from build123d import *

# Parameters (mm, degrees)
BOSS_EXTRUDE1_DEPTH      = 26.67
SKETCH3_W                = 40.639965772
SKETCH3_H                = 26.67
BOSS_EXTRUDE2_DEPTH      = 35.56
CUT_EXTRUDE3_START       = 3.81
CUT_EXTRUDE3_DEPTH       = 19.05
SKETCH9_W                = 30.48
SKETCH9_H                = 19.05
CUT_EXTRUDE4_DEPTH       = 35.533627808
CUT_EXTRUDE8_REACH       = 50.855
SKETCH10_R               = 3.429
SKETCH11_R               = 5.715
CUT_EXTRUDE9_DEPTH       = 3.048
SKETCH12_R               = 5.715
CUT_EXTRUDE10_DEPTH      = 3.048
SKETCH13_R               = 5.715
CUT_EXTRUDE11_DEPTH      = 3.048
CUT_EXTRUDE12_DEPTH      = 49.855187132
CUT_EXTRUDE12_DEPTH_BACK = 49.855187132
SKETCH16_R               = 3.429


with BuildPart() as part:
    # Sketch2 → Boss-Extrude1 (new body)
    with BuildSketch(Plane.XY):
        with BuildLine():
            Line((-20.319982886, 0.026372192), (20.319982886, 0.026372192))
            ThreePointArc((20.319982886, 0.026372192), (0, 20.32), (-20.319982886, 0.026372192))
        make_face()
    extrude(amount=BOSS_EXTRUDE1_DEPTH)

    # Sketch3 → Boss-Extrude2 (add)
    with BuildSketch(Plane(origin=(0, 0.026372192, 0), x_dir=(-1, 0, 0), z_dir=(0, -1, 0))):
        with Locations((0, -13.335)):
            Rectangle(SKETCH3_W, SKETCH3_H)
    extrude(amount=BOSS_EXTRUDE2_DEPTH)

    # Sketch8 → Cut-Extrude3 (cut)
    with BuildSketch(Plane.XY.offset(CUT_EXTRUDE3_START)):
        with BuildLine():
            Line((15.24, 0), (-15.24, 0))
            ThreePointArc((-15.24, 0), (0, 15.24), (15.24, 0))
        make_face()
    extrude(amount=CUT_EXTRUDE3_DEPTH, mode=Mode.SUBTRACT)

    # Sketch9 → Cut-Extrude4 (cut)
    with BuildSketch(Plane(origin=(0, 0, 0), x_dir=(1, 0, 0), z_dir=(0, 1, 0))):
        with Locations((0, -13.335)):
            Rectangle(SKETCH9_W, SKETCH9_H)
    extrude(amount=-CUT_EXTRUDE4_DEPTH, mode=Mode.SUBTRACT)

    # Cut-Extrude8: up to this face of the body (flat: up to its plane)
    cut_extrude8_end = Plane(part.part.faces().sort_by_distance((0, -9.587434333, 26.67))[0])
    # Sketch10 → Cut-Extrude8 (cut, up to the picked face)
    with BuildSketch(Plane.XY, mode=Mode.PRIVATE) as cut_extrude8_sk1:
        with Locations(Location((0, 0, 0), (0, 0, 180))):
            Circle(SKETCH10_R)
    cut_extrude8_tool1 = split(extrude(cut_extrude8_sk1.sketch, amount=CUT_EXTRUDE8_REACH, mode=Mode.PRIVATE), bisect_by=cut_extrude8_end, keep=Keep.BOTH, mode=Mode.PRIVATE)
    add(cut_extrude8_tool1.solids().sort_by(Axis((0, 0, 0), (0, 0, 1)))[0], mode=Mode.SUBTRACT)

    # Sketch11 → Cut-Extrude9 (cut)
    with BuildSketch(Plane.XY):
        with Locations(Location((12.7, 0, 0), (0, 0, 180))):
            Circle(SKETCH11_R)
    extrude(amount=CUT_EXTRUDE9_DEPTH, mode=Mode.SUBTRACT)

    # Sketch12 → Cut-Extrude10 (cut)
    with BuildSketch(Plane.XY):
        with Locations(Location((12.7, -25.4, 0), (0, 0, 180))):
            Circle(SKETCH12_R)
    extrude(amount=CUT_EXTRUDE10_DEPTH, mode=Mode.SUBTRACT)

    # Sketch13 → Cut-Extrude11 (cut)
    with BuildSketch(Plane(origin=(0, 0, 0), x_dir=(-1, 0, 0), z_dir=(0, 0, -1))):
        with Locations((12.7, 0)):
            Circle(SKETCH13_R)
        with Locations((12.7, -25.4)):
            Circle(SKETCH13_R)
    extrude(amount=-CUT_EXTRUDE11_DEPTH, mode=Mode.SUBTRACT)

    # Sketch16 → Cut-Extrude12 (cut, two sides: drawn at the far end of the back side and taken through both)
    with BuildSketch(Plane(origin=(0, 0, 0), x_dir=(-1, 0, 0), z_dir=(0, 0, -1)).offset(-CUT_EXTRUDE12_DEPTH_BACK)):
        with Locations((0, -25.4)):
            Circle(SKETCH16_R)
    extrude(amount=CUT_EXTRUDE12_DEPTH + CUT_EXTRUDE12_DEPTH_BACK, mode=Mode.SUBTRACT)


solid = part.part
Model file for the job. Use its own axes, mm. A direction names the side the tool comes from. Give positions to 0.01 mm unless a question says otherwise; leave off trailing zeros. Loops run counter-clockwise (first coordinate to the right, second up) from the corner with the lowest first, then second, coordinate; pieces in that order, holes last. Notation, with made-up numbers: (82, 13.25) - (109, 13.25) arc R22 cw to (109, 26.25) - close; hole circle Ø3 at (77.25, 61.5). An arc over 180 degrees is marked (long way). Use one line per item in the form item = value.
(1) Cut at A-A (y = -25.4). Give the cut face in (x, z) (3 decimals), then the cut area to 3 significant figures.
Determined:
outline = (-20.32, 0) - (-18.415, 0) - (-18.415, 3.048) - (-6.985, 3.048) - (-6.985, 0) - (-3.429, 0) - (-3.429, 3.81) - (-15.24, 3.81) - (-15.24, 22.86) - (-3.429, 22.86) - (-3.429, 26.67) - (-20.32, 26.67) - close; (3.429, 0) - (6.985, 0) - (6.985, 3.048) - (18.415, 3.048) - (18.415, 0) - (20.32, 0) - (20.32, 26.67) - (3.429, 26.67) - (3.429, 22.86) - (15.24, 22.86) - (15.24, 3.81) - (3.429, 3.81) - close
area = 381 mm^2
(2) Drop flat-ended pins along their axis: P1, Ø4, axis at x = 0, y = -25.4, coming from the +Z side; P2, Ø2, axis at x = 10, z = 9.5, coming from the -Y side; P3, Ø6, axis at x = -3, z = 16.5, coming from the +Y side; P4, Ø6, axis at y = 14.5, z = 9, coming from the -X side. Give the stop position or say it passes through.
Determined:
P1 = through
P2 = 10.55
P3 = 20.32
P4 = -16.75
(3) 3-axis set-ups, long thin cutter, end or side, ignore diameter. For faces 4 (the face through (20.32, -18, 14)), 5 (the face through (0, -10, 22.86)), 6 (the face through (13, -25, 3.048)): which of +Z, -Z, +X, -X, +Y, -Y reach the whole face in a straight line?
Determined:
face_4 = +Z, -Z, +X, +Y, -Y
face_5 = -Y
face_6 = -Z
(4) Pull direction Y, two halves, no side cores. Call faces 1 (the face through (0, -35.534, 25)), 2 (the face through (0, -10, 3.81)), 3 (the face through (0.74, 3.35, 24.74)): pulls with the +Y half, pulls with the -Y half, needs draft (parallel to the pull), parting line crosses it, or undercut.
Determined:
face_1 = pulls with the -Y half
face_2 = needs draft
face_3 = undercut
(5) Cut at C-C (y = -13). Give the cut face in (x, z), then the cut area to 3 significant figures.
Determined:
outline = (-20.32, 0) - (20.32, 0) - (20.32, 26.67) - (-20.32, 26.67) - close; hole (-15.24, 3.81) - (15.24, 3.81) - (15.24, 22.86) - (-15.24, 22.86) - close
area = 503 mm^2
(6) Cut at D-D (z = 2.25). Give the cut face in (x, y) (3 decimals), then the cut area to 3 significant figures.
Determined:
outline = (-20.32, -35.534) - (20.32, -35.534) - (20.32, 0.026) arc R20.32 ccw to (-20.32, 0.026) - close; hole circle Ø11.43 at (-12.7, -25.4); hole circle Ø11.43 at (-12.7, 0); hole circle Ø6.858 at (0, -25.4); hole circle Ø6.858 at (0, 0); hole circle Ø11.43 at (12.7, -25.4); hole circle Ø11.43 at (12.7, 0)
area = 1,610 mm^2
(7) Drill centre lines: L1, parallel to Y at x = 0, z = 1.65; L2, parallel to Z at x = 1, y = -13.5; L3, parallel to Z at x = 10, y = 3. Where is each one in solid material? Low to high.
Determined:
L1 = -35.53 to -28.83, -21.97 to -3.43, 3.43 to 20.32
L2 = 0 to 3.81, 22.86 to 26.67
L3 = 3.05 to 3.81, 22.86 to 26.67
(8) Cut at B-B (x = 0). Give the cut face in (y, z), then the cut area to 3 significant figures.
Determined:
outline = (-35.53, 0) - (-28.83, 0) - (-28.83, 3.81) - (-35.53, 3.81) - close; (-35.53, 22.86) - (-28.83, 22.86) - (-28.83, 26.67) - (-35.53, 26.67) - close; (-21.97, 0) - (-3.43, 0) - (-3.43, 3.81) - (-21.97, 3.81) - close; (-21.97, 22.86) - (-3.43, 22.86) - (-3.43, 26.67) - (-21.97, 26.67) - close; (3.43, 0) - (20.32, 0) - (20.32, 26.67) - (3.43, 26.67) - (3.43, 22.86) - (15.24, 22.86) - (15.24, 3.81) - (3.43, 3.81) - close
area = 418 mm^2
